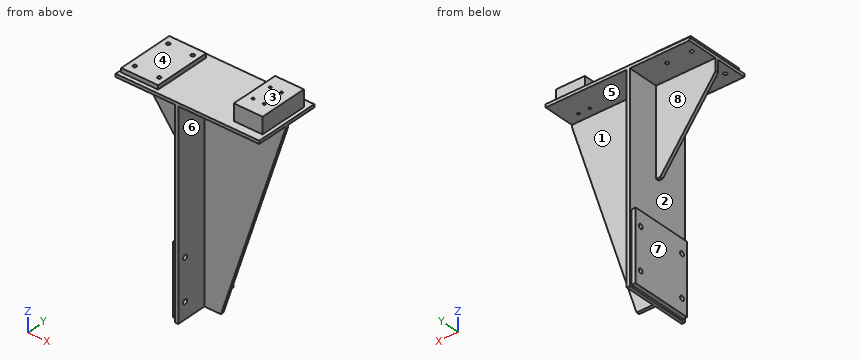
from build123d import *

# Parameters (mm, degrees)
F0_W      = 444.5
F0_H      = 203.2
F1_DEPTH  = 9.525
F2_W      = 114.3
F2_H      = 177.8
F3_DEPTH  = 12.7
F5_D      = 11.1125
F6_W      = 88.9
F6_H      = 152.4
F7_DEPTH  = 50.8
F9_D      = 7.9375
F11_W     = 203.2
F11_H     = 622.3
F12_DEPTH = 9.525
F14_DEPTH = 4.7625
F16_DEPTH = 4.7625
F17_W     = 190.5
F17_H     = 215.9
F18_DEPTH = 12.7
F20_D     = 14.2875


with BuildPart() as f1:
    # F0 (on Top) → F1 (new body)
    with BuildSketch(Plane.XY):
        Rectangle(F0_W, F0_H)
    extrude(amount=-F1_DEPTH)

    # F2 (on face) → F3 (join)
    with BuildSketch(Plane.XY):
        with Locations((-158.75, 0)):
            Rectangle(F2_W, F2_H)
    extrude(amount=F3_DEPTH)

    # F5 (through all)
    with Locations(Plane.XY.offset(12.7)):
        with Locations((-196.85, 61.976), (-120.65, 61.976), (-196.85, -61.976), (-120.65, -61.976)):
            Hole(F5_D / 2)

    # F6 (on face) → F7 (join)
    with BuildSketch(Plane.XY):
        with Locations((166.751, 0)):
            Rectangle(F6_W, F6_H)
    extrude(amount=F7_DEPTH)

    # F9 (through all)
    with Locations(Plane.XY.offset(50.8)):
        with Locations((144.399, 31.75), (179.451, 31.75), (144.399, -31.75), (179.451, -31.75)):
            Hole(F9_D / 2)

    # F11 (on offset) → F12 (join)
    with BuildSketch(Plane(origin=(-38.1, 0, 0), x_dir=(0, -1, 0), z_dir=(-1, 0, 0))):
        with Locations((0, -320.675)):
            Rectangle(F11_W, F11_H)
    extrude(amount=-F12_DEPTH)

    # F13 (on Front) → F14 (join, symmetric)
    with BuildSketch(Plane.XZ):
        Polygon((-38.1, -9.525), (-222.25, -9.525), (-222.25, -47.625), (-50.8, -276.225), (-38.1, -276.225), align=None)
    extrude(amount=F14_DEPTH, both=True)

    # F15 (on Front) → F16 (join, symmetric)
    with BuildSketch(Plane.XZ):
        Polygon((222.25, -9.525), (-28.575, -9.525), (-28.575, -631.825), (22.225, -631.825), (222.25, -15.875), align=None)
    extrude(amount=F16_DEPTH, both=True)

    # F17 (on face) → F18 (join)
    with BuildSketch(Plane(origin=(-38.1, 0, 0), x_dir=(0, -1, 0), z_dir=(-1, 0, 0))):
        with Locations((0, -517.525)):
            Rectangle(F17_W, F17_H)
    extrude(amount=F18_DEPTH)

    # F20 (through all)
    with Locations(Plane(origin=(-50.8, 0, 0), x_dir=(0, -1, 0), z_dir=(-1, 0, 0))):
        with Locations((-76.2, -454.025), (76.2, -454.025), (-76.2, -581.025), (76.2, -581.025)):
            Hole(F20_D / 2)


solid = f1.part
Design review of the part built by this model. Coordinates are the model's own, in mm. Face numbers are marked on the shaded views. A direction names the side the tool comes from. Coordinates: 2 decimals unless noted, no trailing zeros. Order: outer loops, then holes, each group sorted by start corner. A loop starts at its lowest first (then second) coordinate and runs counter-clockwise, first axis right, second up. Notation, with made-up numbers: (-25, -19) -> (14, -19) arc R22 ccw to (14, -12) -> close; hole circle Ø10 at (29.5, 57). An arc over 180 degrees is marked (long way). Use one line per item in the form item = value. Start each with the question number.
(1) Add section D-D on z = -253. State the section outline as (x, y) points (1 decimal).
(2) The part is to be moulded in two halves that separate along Z. For the marked faces 1, 2 and 3, say which applies: +Z half, -Z half, draft (parallel to the pull), parting line (faces both ways), or undercut.
(3) For the marked faces 4, 5, 6, 7 and 8, list the 3-axis set-ups (+Z, -Z, +X, -X, +Y, -Y) from which the entire face can be reached by the end or side of a thin tool; tool diameter is ignored.
(4) Add section B-B on x = -8. State the section outline as (y, z) points (1 decimal), plus the area to 3 significant figures.
(5) Insertion check: pin 1 (1.5 mm diameter, centred on y = 33, z = -332.5, fed in from +X) (3 decimals); pin 2 (12.5 mm diameter, centred on x = 144.399, y = 31.75, fed in from -Z) (3 decimals); pin 3 (4 mm diameter, centred on x = -84.5, z = -117.5, fed in from +Y). Each pin has a flat end and moves straight along its axis. Give the tip position at first contact, or say it passes through.
(6) For probe 1 along Y at (x, z) = (-196.85, 0.25); probe 2 along Z at (x, y) = (-45, -76) (3 decimals); probe 3 along Y at (x, z) = (181, 4.5), list the stretches that pass through material, from the lowest coordinate up.
(7) Add section A-A on y = -12.5. State the section outline as (x, z) points (3 decimals).
Answer block:
q1.outline = (-68.2, -4.8) -> (-38.1, -4.8) -> (-38.1, -101.6) -> (-28.6, -101.6) -> (-28.6, -4.8) -> (145.2, -4.8) -> (145.2, 4.8) -> (-28.6, 4.8) -> (-28.6, 101.6) -> (-38.1, 101.6) -> (-38.1, 4.8) -> (-68.2, 4.8) -> close
q2.face_1 = draft
q2.face_2 = undercut
q2.face_3 = +Z half
q3.face_4 = +Z, -X, +Y, -Y
q3.face_5 = -Z, +X, +Y
q3.face_6 = -Z, +X, -Y
q3.face_7 = -Z, -X, +Y, -Y
q3.face_8 = -X, +Y
q4.outline = (-101.6, -9.5) -> (-4.8, -9.5) -> (-4.8, -631.8) -> (4.8, -631.8) -> (4.8, -9.5) -> (101.6, -9.5) -> (101.6, 0) -> (-101.6, 0) -> close
q4.area = 7,860 mm²
q5.pin_1 = -28.575
q5.pin_2 = -9.525
q5.pin_3 = 4.76
q6.probe_1 = -88.9 to -67.53, -56.42 to 56.42, 67.53 to 88.9
q6.probe_2 = -625.475 to -588.166, -573.884 to -461.166, -446.884 to -409.575, -9.525 to 0
q6.probe_3 = -76.2 to -35.4, -28.1 to 28.1, 35.4 to 76.2
q7.outline = (-222.25, -9.525) -> (-38.1, -9.525) -> (-38.1, -409.575) -> (-50.8, -409.575) -> (-50.8, -625.475) -> (-38.1, -625.475) -> (-38.1, -631.825) -> (-28.575, -631.825) -> (-28.575, -9.525) -> (222.25, -9.525) -> (222.25, 0) -> (211.201, 0) -> (211.201, 50.8) -> (122.301, 50.8) -> (122.301, 0) -> (-101.6, 0) -> (-101.6, 12.7) -> (-215.9, 12.7) -> (-215.9, 0) -> (-222.25, 0) -> close
